```python
from build123d import *

# Parameters (mm, degrees)
F2_DEPTH    = 520
F2_TAPER    = 2
F3_T1_DEPTH = 701.1716597564
F4_R        = 10
F5_T        = -2.5


# Not quite as in the source:
# - a fillet or chamfer that OpenCascade refuses, or shapes differently, is made with other operations: its cross-section is extruded or revolved along the edge and cut away or added


with BuildPart() as f2:
    # F0 (on Top) → F2 (new body)
    with BuildSketch(Plane.XY):
        Polygon((120, 120), (0, 120), (60, 60), align=None)
        Polygon((60, 60), (120, 0), (120, 120), align=None)
        Polygon((60, 60), (0, 0), (120, 0), align=None)
        Polygon((0, 120), (0, 0), (60, 60), align=None)
    extrude(amount=F2_DEPTH, taper=F2_TAPER)

    # F3: chamfer of 120 on 1 edges, made by hand

    # F3_s2 → F3_t1 (cut)
    with BuildSketch(Plane.XZ.offset(-410.5858298782)):
        Polygon((13.9708605314, 400.0731007577), (138.1588001357, 520), (18.1588001357, 520), align=None)
    extrude(amount=F3_T1_DEPTH, mode=Mode.SUBTRACT)

    # F4
    f4_edges = [f2.edges().sort_by_distance(p)[0] for p in [
        (6.98543, 6.98543, 200.03655),
        (6.98543, 113.01457, 200.03655),
        (111.512985, 8.487015, 243.03631),
        (111.512985, 111.512985, 243.03631),
    ]]
    fillet(f4_edges, radius=F4_R)

    # F5
    f5_openings = [f2.faces().sort_by_distance(p)[0] for p in [
        (60, 60, 0),
    ]]
    offset(amount=F5_T, openings=f5_openings)


solid = f2.part
```
Design review of the part built by this model. Coordinates are the model's own, in mm. A direction names the side the tool comes from. Coordinates: 2 decimals unless noted, no trailing zeros. Order: outer loops, then holes, each group sorted by start corner. A loop starts at its lowest first (then second) coordinate and runs counter-clockwise, first axis right, second up.
1) For faces 4 (the cylindrical face through (108.39, 108.54, 246.48)), 5 (the cylindrical face through (106.739, 106.855, 243.596)), list the 3-axis set-ups (+Z, -Z, +X, -X, +Y, -Y) from which the entire face can be reached by the end or side of a thin tool; tool diameter is ignored.
2) Mouldability with a two-part tool opening along Y and no side actions: class faces 1 (the cylindrical face through (10.11, 10.27, 207.95)), 2 (the flat face through (57.989, 60.606, 439.105)), 3 (the cylindrical face through (10.27, 109.89, 207.95)) as +Y half, -Y half, draft (parallel to the pull), parting line (faces both ways), or undercut.
3) Take a section at A-A, the plane x = 58. Give the boundary of the cut face in (y, z), and give its area (3 significant figures).
4) Wall thickness on line 1 along X through (y, z) = (89.5, 149); line 2 along X through (y, z) = (29, 460); line 3 along Y through (x, z) = (95, 299): over which ranges is each line inside the solid? List them lowest first.
5) Clearance check with flat-ended pins moving along their axes: pin 1 (3 mm diameter, centred on x = 34, z = 345.5, fed in from +Y); pin 2 (12 mm diameter, centred on x = 60, y = 44, fed in from -Z); pin 3 (2 mm diameter, centred on x = 76.5, z = 416.5, fed in from -Y). State where each tip first meets the part, or that it passes through.
6) Take a section at B-B, the plane y = 51. Give the boundary of the cut face in (x, z).
Returned:
1. face 4: +Z, +X, +Y
1. face 5: -Z
2. face 1: -Y half
2. face 2: undercut
2. face 3: +Y half
3. outline: (0, 0) - (2.5, 0) - (17.84, 439.12) - (102.16, 439.12) - (117.5, 0) - (120, 0) - (104.54, 442.59) - (15.46, 442.59) - close
3. area: 2,510 mm2
4. line 1: x = 5.2 to 7.7, 112.3 to 114.8
4. line 2: x = 76.03 to 79.63, 101.43 to 103.94
4. line 3: y = 10.44 to 12.94, 107.06 to 109.56
5. pin 1: stops at y = 107.99
5. pin 2: stops at z = 435.25
5. pin 3: stops at y = 14.51
6. outline: (0, 0) - (2.5, 0) - (16.43, 398.98) - (100.72, 480.37) - (117.5, 0) - (120, 0) - (103.03, 486.07) - (13.97, 400.07) - close
